Geometry check sheet. Reference: the model listing, model coordinates, mm. Coordinates: 2 decimals unless noted, no trailing zeros. Write each loop counter-clockwise with the first axis right and the second up, starting at its lowest first coordinate (ties: lowest second). Pieces come first, ordered by that corner, then holes. Notation, with made-up numbers: (-31, 1.5) -> (26, 1.5) arc R26 ccw to (26, 29.5) -> close; hole circle Ø11 at (9.25, -34). An arc over 180 degrees is marked (long way). Use a Markdown table: item, result.
Autodesk Inventor part; units mm, degrees
ref_plane "YZ Plane" through (0, 0, 0) normal (1, 0, 0) x (0, 1, 0)
ref_plane "XZ Plane" through (0, 0, 0) normal (0, 1, 0) x (-1, 0, 0)
ref_plane "XY Plane" through (0, 0, 0) normal (0, 0, 1) x (1, 0, 0)
sketch "Sketch1" plane through (0, 0, 0) normal (0, 0, 1) x (1, 0, 0)
  line L0 (44.8, 3.5) -> (44.8, 89.5) construction
  line L1 (-45, 89.5) -> (44.8, 89.5) construction
  line L2 (-45, 94.5) -> (-45, 89.5) construction
  line L3 (-50, 92.5) -> (-45, 94.5) construction
  line L4 (-50, 0.5) -> (-50, 92.5) construction
  line L5 (-45, -1.5) -> (-50, 0.5) construction
  line L6 (-45, 3.5) -> (-45, -1.5) construction
  line L7 (44.8, 3.5) -> (-45, 3.5) construction
  line L8 (-49.9, 92.4323) -> (-45.1, 94.3523)
  line L9 (-45.1, 94.3523) -> (-45.1, 89.4)
  line L10 (-45.1, 89.4) -> (44.7, 89.4) construction
  line L11 (44.7, 89.4) -> (44.7, 3.6) construction
  line L12 (44.7, 3.6) -> (-45.1, 3.6) construction
  line L13 (-45.1, 3.6) -> (-45.1, -1.3523)
  line L14 (-45.1, -1.3523) -> (-49.9, 0.5677)
  line L15 (-49.9, 0.5677) -> (-49.9, 92.4323)
  line L16 (-45.1, 89.4) -> (-45.1, 3.6)
  point P0 (0, 0)
  dimension "d0" = 0.1
extrude "Extrusion1" add sketch "Sketch1" against normal blind 100
sketch "Sketch2" plane through (-49.9, 0.5677, -100) normal (-0.3713907, -0.9284767, 0) x (0.9284767, -0.3713907, 0)
  circle A0 centre (2.5849, 10) radius 1
  line L0 (5.1698, 0) -> (0, 0)
  line L1 (2.5849, 0) -> (2.5849, 10) construction
  point P0 (46.5418, 100)
  dimension "d3" = 2
  dimension "d4" = 10
extrude "Extrusion2" add sketch "Sketch2" along normal blind 0.7
fillet "Fillet1" radius 1 2 edges at (-48.6885, -0.6708, -90) (-48.4285, -0.0209, -90)
properties part number "door2" material "ABS Plastic"
Item 1: Thickness scan on L1, parallel to Y at x = -48.45, z = -16.5; L2, parallel to Y at x = -47.4, z = -54. Record the ranges inside material, lowest first. Write a range as [from, to].
Answer block:
| item | result |
|---|---|
| L1 | y = [-0.01, 93.01] |
| L2 | y = [-0.43, 93.43] |
Item 2: Section check A-A on z = -86. Record the boundary of the cut face in (x, y), then the cut area to 3 significant figures.
Answer block:
| item | result |
|---|---|
| outline | (-49.9, 0.57) -> (-45.1, -1.35) -> (-45.1, 94.35) -> (-49.9, 92.43) -> close |
| area | 450 mm^2 |
Item 3: Depth check by flat-ended pin: P1, Ø1.5, axis at x = -47.5, z = -40, coming from the +Y side. Enter the tip coordinate at first touch or a pass-through.
Answer block:
| item | result |
|---|---|
| P1 | stops at y = 93.69 |
